Can you work these out from the model? Positions are in its coordinate system, mm. Face numbers are marked on the shaded views. A direction names the side the tool comes from. Coordinates: 2 decimals unless noted, no trailing zeros. Loops run counter-clockwise (first coordinate to the right, second up) from the corner with the lowest first, then second, coordinate; pieces in that order, holes last. Notation, with made-up numbers: (-14.5, 41.5) - (-4.5, 41.5) arc R11 ccw to (-4.5, 53.5) - close; hole circle Ø5 at (20, 78.5). An arc over 180 degrees is marked (long way). Put each result on its own line as item: value. Start each with the question number.
from build123d import *

# Parameters (mm, degrees)
ESQUISSE1_W                = 400
ESQUISSE1_H                = 120
BOSS_EXTRU_1_DEPTH         = 100
ESQUISSE2_W                = 380
ESQUISSE2_H                = 100
ENL_V_MAT_EXTRU_1_DEPTH    = 90
ESQUISSE3_W                = 120
ESQUISSE3_H                = 80
BOSS_EXTRU_2_DEPTH         = 60
ESQUISSE4_W                = 90
ESQUISSE4_H                = 50
BOSS_EXTRU_3_DEPTH         = 20
ESQUISSE5_W                = 60
ESQUISSE5_H                = 20
BOSS_EXTRU_4_DEPTH         = 20
ESQUISSE9_W                = 50
ESQUISSE9_H                = 10
ENL_V_MAT_EXTRU_3_DEPTH    = 10
R_P_TITION_LIN_AIRE1_COUNT = 5
R_P_TITION_LIN_AIRE1_PITCH = 80


with BuildPart() as part:
    # Esquisse1 → Boss.-Extru.1 (new body)
    with BuildSketch(Plane(origin=(0, 0, 0), x_dir=(1, 0, 0), z_dir=(0, 1, 0))):
        with Locations((200, 60)):
            Rectangle(ESQUISSE1_W, ESQUISSE1_H)
    extrude(amount=BOSS_EXTRU_1_DEPTH)

    # Esquisse2 → Enlèv. mat.-Extru.1 (cut)
    with BuildSketch(Plane(origin=(0, 100, 0), x_dir=(1, 0, 0), z_dir=(0, 1, 0))):
        with Locations((200, 60)):
            Rectangle(ESQUISSE2_W, ESQUISSE2_H)
    extrude(amount=-ENL_V_MAT_EXTRU_1_DEPTH, mode=Mode.SUBTRACT)

    # Esquisse3 → Boss.-Extru.2 (add)
    with BuildSketch(Plane(origin=(0, 10, 0), x_dir=(1, 0, 0), z_dir=(0, 1, 0))):
        with Locations((80, 60)):
            Rectangle(ESQUISSE3_W, ESQUISSE3_H)
    extrude(amount=BOSS_EXTRU_2_DEPTH)

    # Esquisse4 → Boss.-Extru.3 (add)
    with BuildSketch(Plane(origin=(0, 10, 0), x_dir=(1, 0, 0), z_dir=(0, 1, 0))):
        with Locations((215, 60)):
            Rectangle(ESQUISSE4_W, ESQUISSE4_H)
    extrude(amount=BOSS_EXTRU_3_DEPTH)

    # Esquisse5 → Boss.-Extru.4 (add)
    with BuildSketch(Plane(origin=(0, 10, 0), x_dir=(1, 0, 0), z_dir=(0, 1, 0))):
        with Locations((320, 60)):
            Rectangle(ESQUISSE5_W, ESQUISSE5_H)
    extrude(amount=BOSS_EXTRU_4_DEPTH)

    # Esquisse9 → Enlèv. mat.-Extru.3 (cut)
    with BuildSketch(Plane(origin=(0, 0, -120), x_dir=(-1, 0, 0), z_dir=(0, 0, -1))):
        with Locations((-360, 20)):
            Rectangle(ESQUISSE9_W, ESQUISSE9_H)
    enl_v_mat_extru_3 = extrude(amount=-ENL_V_MAT_EXTRU_3_DEPTH, mode=Mode.SUBTRACT)

    # Répétition linéaire1: Enlèv. mat.-Extru.3 ×5
    with Locations(*[(-i * R_P_TITION_LIN_AIRE1_PITCH, 0, 0) for i in range(1, R_P_TITION_LIN_AIRE1_COUNT)]):
        add(enl_v_mat_extru_3, mode=Mode.SUBTRACT)


solid = part.part
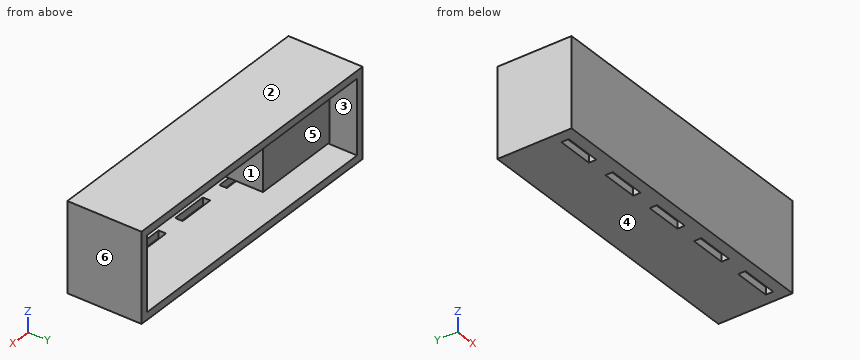
Q1. I want a section at D-D on x = 91. List the corners of the cut face in (y, z) for me, and give its area (3 significant figures).
Q2. Will these pins go through, and if not, where does the flat tip stop? pin 1 (1.5 mm diameter, centred on x = 194.5, z = -107.5, fed in from +Y); pin 2 (16 mm diameter, centred on x = 318, z = -56.5, fed in from +Y); pin 3 (24 mm diameter, centred on x = 98.5, z = -43.5, fed in from +Y).
Q3. On a 3-axis mill with a long thin cutter (end or side, diameter ignored), from which of +Z, -Z, +X, -X, +Y, -Y can I reach the whole of each face in a straight line? I mean the marked faces 5 and 6. Say none if no direction works.
Q4. I want a section at B-B on x = 295. List the corners of the cut face in (y, z) for me.
Q5. We'd pull the mould along Z, two halves only. Please class the marked faces 1, 2, 3 and 4: released by +Z, released by -Z, zero draft, split by the parting line, or undercut.
Q6. I want a section at C-C on z = -77.5. List the corners of the cut face in (x, y) for me.
Q7. I want a section at A-A on y = 64. List the corners of the cut face in (x, z) for me, and give its area (3 significant figures).
Q8. Please list where these lines run through material, in increasing order: line 1 along X through (y, z) = (19.5, -76); line 2 along X through (y, z) = (30.5, -27); line 3 along X through (y, z) = (24.5, -61). Write a range as [from, to].
Calculated:
1. outline: (0, -120) - (100, -120) - (100, -110) - (10, -110) - (10, -100) - (70, -100) - (70, -20) - (10, -20) - (10, -10) - (100, -10) - (100, 0) - (0, 0) - close
1. area: 7,800 mm2
2. pin 1: y = 10
2. pin 2: y = 30
2. pin 3: y = 70
3. face 5: +Y
3. face 6: +Z, -Z, +X, +Y, -Y
4. outline: (0, -120) - (15, -120) - (15, -110) - (10, -110) - (10, -70) - (30, -70) - (30, -50) - (10, -50) - (10, -10) - (100, -10) - (100, 0) - (0, 0) - close; (25, -120) - (100, -120) - (100, -110) - (25, -110) - close
5. face 1: undercut
5. face 2: released by +Z
5. face 3: undercut
5. face 4: released by -Z
6. outline: (0, 0) - (400, 0) - (400, 100) - (390, 100) - (390, 10) - (260, 10) - (260, 30) - (170, 30) - (170, 10) - (140, 10) - (140, 70) - (20, 70) - (20, 10) - (10, 10) - (10, 100) - (0, 100) - close
7. outline: (0, -120) - (400, -120) - (400, 0) - (0, 0) - close; (20, -100) - (140, -100) - (140, -20) - (20, -20) - close; hole (10, -110) - (390, -110) - (390, -10) - (10, -10) - close
7. area: 19,600 mm2
8. line 1: [0, 10], [20, 140], [170, 260], [390, 400]
8. line 2: [0, 10], [20, 140], [390, 400]
8. line 3: [0, 10], [20, 140], [170, 260], [290, 350], [390, 400]
